```python
from build123d import *

# Parameters (mm, degrees)
F0_R     = 10.922
F1_DEPTH = 7


with BuildPart() as f1:
    # F0 (on Top) → F1 (new body)
    with BuildSketch(Plane.XY):
        with BuildLine():
            ThreePointArc((-39.3408468404, -11.8787395478), (-24.9781006693, -12.3639309467), (-17.653, 0))
            ThreePointArc((-17.653, 0), (-18.8994874853, 5.7956653725), (-22.4185156572, 10.5664))
            ThreePointArc((-22.4185156572, 10.5664), (-42.3164, 9.3314843428), (-41.0814843428, -10.5664))
            ThreePointArc((-41.0814843428, -10.5664), (-40.2200100529, -11.2343007326), (-39.3408468404, -11.8787395478))
        make_face()
        with Locations((-31.75, 0)):
            Circle(F0_R, mode=Mode.SUBTRACT)
        with BuildLine():
            Line((-17.653, 0), (-14.097, 0))
            ThreePointArc((-14.097, 0), (-12.848539058, 5.800039058), (-9.324289058, 10.57275))
            ThreePointArc((-9.324289058, 10.57275), (-15.8705493616, 8.8106264002), (-22.4185156572, 10.5664))
            ThreePointArc((-22.4185156572, 10.5664), (-18.8994874853, 5.7956653725), (-17.653, 0))
        make_face()
        with BuildLine():
            ThreePointArc((7.5908468404, -11.8787395478), (-6.7718993307, -12.3639309467), (-14.097, 0))
            Line((-14.097, 0), (-17.653, 0))
            ThreePointArc((-17.653, 0), (-24.9781006693, -12.3639309467), (-39.3408468404, -11.8787395478))
            ThreePointArc((-39.3408468404, -11.8787395478), (-15.875, -19.383375), (7.5908468404, -11.8787395478))
        make_face()
        with BuildLine():
            Line((14.097, 0), (10.922, 0))
            ThreePointArc((10.922, 0), (0, -10.922), (-10.922, 0))
            Line((-10.922, 0), (-14.097, 0))
            ThreePointArc((-14.097, 0), (-6.7718993307, -12.3639309467), (7.5908468404, -11.8787395478))
            ThreePointArc((7.5908468404, -11.8787395478), (8.4700100529, -11.2343007326), (9.3314843428, -10.5664))
            ThreePointArc((9.3314843428, -10.5664), (12.8505125147, -5.7956653725), (14.097, 0))
        make_face()
        with BuildLine():
            ThreePointArc((-10.922, 0), (0, 10.922), (10.922, 0))
            Line((10.922, 0), (14.097, 0))
            ThreePointArc((14.097, 0), (6.7722595018, 12.3637336691), (-7.5901547478, 11.879181786))
            ThreePointArc((-7.5901547478, 11.879181786), (-8.4659884875, 11.2376025013), (-9.324289058, 10.57275))
            ThreePointArc((-9.324289058, 10.57275), (-12.848539058, 5.800039058), (-14.097, 0))
            Line((-14.097, 0), (-10.922, 0))
        make_face()
        with BuildLine():
            ThreePointArc((-7.5901547478, 11.879181786), (6.7722595018, 12.3637336691), (14.097, 0))
            Line((14.097, 0), (17.653, 0))
            ThreePointArc((17.653, 0), (24.9738232973, 12.3615872077), (39.3326252102, 11.8839893942))
            ThreePointArc((39.3326252102, 11.8839893942), (15.8704669391, 19.3801997895), (-7.5901547478, 11.879181786))
        make_face()
        with BuildLine():
            Line((17.653, 0), (14.097, 0))
            ThreePointArc((14.097, 0), (12.8505125147, -5.7956653725), (9.3314843428, -10.5664))
            ThreePointArc((9.3314843428, -10.5664), (15.875, -8.8138), (22.4185156572, -10.5664))
            ThreePointArc((22.4185156572, -10.5664), (18.8994874853, -5.7956653725), (17.653, 0))
        make_face()
        with BuildLine():
            ThreePointArc((39.3326252102, 11.8839893942), (24.9738232973, 12.3615872077), (17.653, 0))
            ThreePointArc((17.653, 0), (18.8994874853, -5.7956653725), (22.4185156572, -10.5664))
            ThreePointArc((22.4185156572, -10.5664), (37.5456653725, -12.8505125147), (45.847, 0))
            ThreePointArc((45.847, 0), (44.6005125147, 5.7956653725), (41.0814843428, 10.5664))
            ThreePointArc((41.0814843428, 10.5664), (40.2159714919, 11.2370300074), (39.3326252102, 11.8839893942))
        make_face()
        with BuildLine():
            ThreePointArc((42.672, 0), (31.75, -10.922), (20.828, 0))
            ThreePointArc((20.828, 0), (31.75, 10.922), (42.672, 0))
        make_face(mode=Mode.SUBTRACT)
    extrude(amount=F1_DEPTH)


solid = f1.part
```
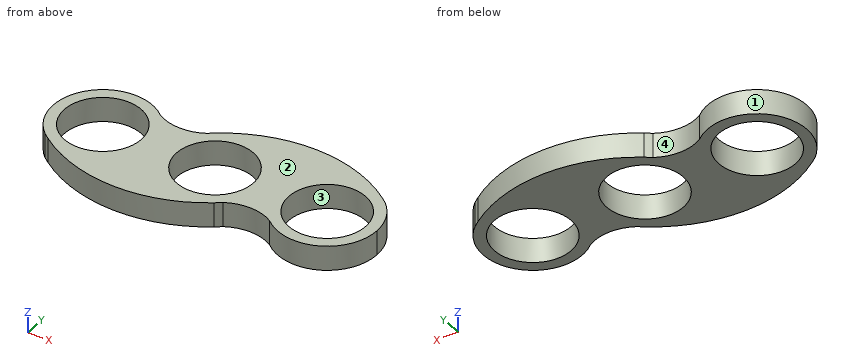
Verification items for the finished model (mm, model axes). Face numbers are marked on the shaded views. Round coordinates to 2 decimals unless told otherwise and drop trailing zeros. Write each loop counter-clockwise with the first axis right and the second up, starting at its lowest first coordinate (ties: lowest second). Pieces come first, ordered by that corner, then holes. Notation, with made-up numbers: (43.5, 57) - (78.5, 57) arc R10 cw to (78.5, 67) - close; hole circle Ø7 at (-13, 37.25). An arc over 180 degrees is marked (long way). Answer as a JSON object with one key per item and string values. Group by question number.
Q1. Section check B-B, the plane y = 5. Enter the section's corners in (x, z).
Q2. Section check C-C, the plane x = 31.75. Enter the section's corners in (y, z), plus the area to 3 significant figures.
Q3. Thickness scan on line 1 (X direction, y = 5.5, z = 3.75); line 2 (X direction, y = -8, z = 0.75); line 3 (X direction, y = 12.5, z = 2.5). Record the ranges inside material, lowest first.
Q4. Mould release check, pull along Y, two halves, no side actions. Record for the marked faces 1, 2, 3 and 4: released by +Y, released by -Y, zero draft, split by the parting line, or undercut.
Q5. Section check D-D, the plane x = -25. Enter the section's corners in (y, z).
Q6. Section check A-A, the plane z = 6. Give the number of separate pieces and of enclosed holes in the cut face, plus the area to 3 significant figures.
Q7. Go/stop test with flat-tipped pins: pin 1 Ø2 at (y, z) = (3, 4.5) entering from -X; pin 2 Ø1 at (x, z) = (-24.5, 3.5) entering from +Y; pin 3 Ø3 at (y, z) = (-10, 2) entering from -X. Record where each tip stops, or that it passes through.
Found:
{
 "1": {"outline": "(-44.93, 0) - (-41.46, 0) - (-41.46, 7) - (-44.93, 7) - close; (-22.04, 0) - (-9.71, 0) - (-9.71, 7) - (-22.04, 7) - close; (9.71, 0) - (22.04, 0) - (22.04, 7) - (9.71, 7) - close; (41.46, 0) - (44.93, 0) - (44.93, 7) - (41.46, 7) - close"},
 "2": {"outline": "(-14.1, 0) - (-10.92, 0) - (-10.92, 7) - (-14.1, 7) - close; (10.92, 0) - (16.13, 0) - (16.13, 7) - (10.92, 7) - close", "area": "58.7 mm^2"},
 "3": {"line 1": "x = -44.73 to -41.19, -22.31 to -9.44, 9.44 to 22.31, 41.19 to 44.73", "line 2": "x = -43.36 to -39.19, -24.31 to -7.44, 7.44 to 24.31, 39.19 to 43.36", "line 3": "x = -38.27 to -25.23, -6.69 to 38.44"},
 "4": {"face 1": "split by the parting line", "face 2": "zero draft", "face 3": "undercut", "face 4": "released by +Y"},
 "5": {"outline": "(-18.34, 0) - (-8.59, 0) - (-8.59, 7) - (-18.34, 7) - close; (8.59, 0) - (12.38, 0) - (12.38, 7) - (8.59, 7) - close"},
 "6": {"separate pieces": "1", "enclosed holes": "3", "area": "1,420 mm^2"},
 "7": {"pin 1": "stops at x = -45.7", "pin 2": "stops at y = 12.38", "pin 3": "stops at x = -43"}
}
